from build123d import *

# Parameters (mm, degrees)
F1_DEPTH = 30
F0_R     = 2
F2_DEPTH = 5


with BuildPart() as f1:
    # F0 (on Front) → F1 (new body)
    with BuildSketch(Plane.XZ):
        with BuildLine():
            ThreePointArc((-22.7745900685, 10.3110643104), (0, 25), (22.7745900685, 10.3110643104))
            Line((22.7745900685, 10.3110643104), (28.1723615053, 10.3110643104))
            ThreePointArc((28.1723615053, 10.3110643104), (0, 30), (-28.1723615053, 10.3110643104))
            Line((-28.1723615053, 10.3110643104), (-22.7745900685, 10.3110643104))
        make_face()
        with BuildLine():
            Line((28.1723615053, -10.3110643104), (22.7745900685, -10.3110643104))
            ThreePointArc((22.7745900685, -10.3110643104), (0, -25), (-22.7745900685, -10.3110643104))
            Line((-22.7745900685, -10.3110643104), (-28.1723615053, -10.3110643104))
            ThreePointArc((-28.1723615053, -10.3110643104), (0, -30), (28.1723615053, -10.3110643104))
        make_face()
        with BuildLine():
            ThreePointArc((-22.7745900685, -10.3110643104), (-25, 0), (-22.7745900685, 10.3110643104))
            Line((-22.7745900685, 10.3110643104), (-28.1723615053, 10.3110643104))
            ThreePointArc((-28.1723615053, 10.3110643104), (-30, 0), (-28.1723615053, -10.3110643104))
            Line((-28.1723615053, -10.3110643104), (-22.7745900685, -10.3110643104))
        make_face()
        with BuildLine():
            ThreePointArc((22.7745900685, 10.3110643104), (24.4373152342, 5.2742415705), (25, 0))
            ThreePointArc((25, 0), (24.4373152342, -5.2742415705), (22.7745900685, -10.3110643104))
            Line((22.7745900685, -10.3110643104), (28.1723615053, -10.3110643104))
            ThreePointArc((28.1723615053, -10.3110643104), (29.5395569124, -5.2358931826), (30, 0))
            ThreePointArc((30, 0), (29.5395569124, 5.2358931826), (28.1723615053, 10.3110643104))
            Line((28.1723615053, 10.3110643104), (22.7745900685, 10.3110643104))
        make_face()
    extrude(amount=F1_DEPTH)

    # F0 (on Front) → F2 (join)
    with BuildSketch(Plane.XZ):
        with BuildLine():
            ThreePointArc((-28.1723615053, -10.3110643104), (-30, 0), (-28.1723615053, 10.3110643104))
            Line((-28.1723615053, 10.3110643104), (-33.4467031677, 10.3110643104))
            ThreePointArc((-33.4467031677, 10.3110643104), (-35, 0), (-33.4467031677, -10.3110643104))
            Line((-33.4467031677, -10.3110643104), (-28.1723615053, -10.3110643104))
        make_face()
        with BuildLine():
            ThreePointArc((-28.1723615053, 10.3110643104), (0, 30), (28.1723615053, 10.3110643104))
            Line((28.1723615053, 10.3110643104), (33.4467031677, 10.3110643104))
            ThreePointArc((33.4467031677, 10.3110643104), (0, 35), (-33.4467031677, 10.3110643104))
            Line((-33.4467031677, 10.3110643104), (-28.1723615053, 10.3110643104))
        make_face()
        with BuildLine():
            Line((33.4467031677, 10.3110643104), (28.1723615053, 10.3110643104))
            ThreePointArc((28.1723615053, 10.3110643104), (29.5395569124, 5.2358931826), (30, 0))
            ThreePointArc((30, 0), (29.5395569124, -5.2358931826), (28.1723615053, -10.3110643104))
            Line((28.1723615053, -10.3110643104), (33.4467031677, -10.3110643104))
            ThreePointArc((33.4467031677, -10.3110643104), (34.60949733, -5.2137025774), (35, 0))
            ThreePointArc((35, 0), (34.60949733, 5.2137025774), (33.4467031677, 10.3110643104))
        make_face()
        with BuildLine():
            Line((33.4467031677, -10.3110643104), (28.1723615053, -10.3110643104))
            ThreePointArc((28.1723615053, -10.3110643104), (0, -30), (-28.1723615053, -10.3110643104))
            Line((-28.1723615053, -10.3110643104), (-33.4467031677, -10.3110643104))
            ThreePointArc((-33.4467031677, -10.3110643104), (0, -35), (33.4467031677, -10.3110643104))
        make_face()
        with BuildLine():
            ThreePointArc((-33.4467031677, -10.3110643104), (-35, 0), (-33.4467031677, 10.3110643104))
            Line((-33.4467031677, 10.3110643104), (-46.3196326792, 10.3110643104))
            ThreePointArc((-46.3196326792, 10.3110643104), (-49.8551665852, 8.8465982163), (-51.3196326792, 5.3110643104))
            Line((-51.3196326792, 5.3110643104), (-51.3196326792, -5.3110643104))
            ThreePointArc((-51.3196326792, -5.3110643104), (-49.8551665852, -8.8465982163), (-46.3196326792, -10.3110643104))
            Line((-46.3196326792, -10.3110643104), (-33.4467031677, -10.3110643104))
        make_face()
        with Locations((-43.3196326792, 0)):
            Circle(F0_R, mode=Mode.SUBTRACT)
        with BuildLine():
            Line((46.3196326792, 10.3110643104), (33.4467031677, 10.3110643104))
            ThreePointArc((33.4467031677, 10.3110643104), (34.60949733, 5.2137025774), (35, 0))
            ThreePointArc((35, 0), (34.60949733, -5.2137025774), (33.4467031677, -10.3110643104))
            Line((33.4467031677, -10.3110643104), (46.3196326792, -10.3110643104))
            ThreePointArc((46.3196326792, -10.3110643104), (49.8551665852, -8.8465982163), (51.3196326792, -5.3110643104))
            Line((51.3196326792, -5.3110643104), (51.3196326792, 5.3110643104))
            ThreePointArc((51.3196326792, 5.3110643104), (49.8551665852, 8.8465982163), (46.3196326792, 10.3110643104))
        make_face()
        with Locations((43.3196326792, 0)):
            Circle(F0_R, mode=Mode.SUBTRACT)
    extrude(amount=F2_DEPTH)


solid = f1.part
Verification items for the finished model (mm, model axes). A direction names the side the tool comes from. Coordinates: 2 decimals unless noted, no trailing zeros. Order: outer loops, then holes, each group sorted by start corner. A loop starts at its lowest first (then second) coordinate and runs counter-clockwise, first axis right, second up.
1. Set-up check for faces 1 (the face through (40, -2, 10.311)), 2 (the face through (-40, -2, -10.311)), 3 (the face through (-15.4, -5, 26.1)), 4 (the face through (-40, -2, 10.311)), 5 (the face through (40, -2, -10.311)): record each of +Z, -Z, +X, -X, +Y, -Y from which the full face is reachable in a straight line by a thin tool's end or side.
Results found:
face 1: +Z, +X, +Y, -Y
face 2: -Z, -X, +Y, -Y
face 3: -Y
face 4: +Z, -X, +Y, -Y
face 5: -Z, +X, +Y, -Y
2. Sectioned sample at A-A, the plane y = -15.25. Record the cut outline in (x, z).
Results found:
outline: circle Ø60 at (0, 0); hole circle Ø50 at (0, 0)
3. Release check for a two-part mould opening along X. For faces 6 (the face through (-45.318, -2.465, 0.088)), 7 (the face through (-0.623, -2.465, -34.994)), 8 (the face through (-23, 0, 11)), 9 (the face through (45.167, -2.465, -0.766)) record: +X half, -X half, draft (parallel to the pull), parting line (faces both ways), or undercut.
Results found:
face 6: undercut
face 7: parting line
face 8: draft
face 9: undercut
4. Go/stop test with flat-tipped pins: pin 1 Ø1.5 at (x, y) = (40, -3.5) entering from -Z; pin 2 Ø3 at (x, z) = (16.5, -16.5) entering from -Y (3 decimals); pin 3 Ø8 at (y, z) = (-21, 22.5) entering from +X; pin 4 Ø12 at (x, y) = (-24.5, -18.5) entering from -Z. Record where each tip stops, or that it passes through.
Results found:
pin 1: stops at z = -10.31
pin 2: passes through
pin 3: stops at x = 23.62
pin 4: stops at z = -23.62
5. Sectioned sample at C-C, the plane y = -3. Record the cut outline in (x, z), and give its area (3 significant figures).
Results found:
outline: (-51.32, -5.31) arc R5 ccw to (-46.32, -10.31) - (-33.45, -10.31) arc R35 ccw to (33.45, -10.31) - (46.32, -10.31) arc R5 ccw to (51.32, -5.31) - (51.32, 5.31) arc R5 ccw to (46.32, 10.31) - (33.45, 10.31) arc R35 ccw to (-33.45, 10.31) - (-46.32, 10.31) arc R5 ccw to (-51.32, 5.31) - close; hole circle Ø4 at (-43.32, 0); hole circle Ø50 at (0, 0); hole circle Ø4 at (43.32, 0)
area: 2,530 mm2
6. Sectioned sample at D-D, the plane z = 21. Record the cut outline in (x, y), and give its area (3 significant figures).
Results found:
outline: (-28, -5) - (-21.42, -5) - (-21.42, -30) - (-13.56, -30) - (-13.56, 0) - (-28, 0) - close; (13.56, -30) - (21.42, -30) - (21.42, -5) - (28, -5) - (28, 0) - (13.56, 0) - close
area: 537 mm2
7. Sectioned sample at B-B, the plane x = -14.5. Record the cut outline in (y, z).
Results found:
outline: (-30, -26.26) - (-5, -26.26) - (-5, -31.86) - (0, -31.86) - (0, -20.37) - (-30, -20.37) - close; (-30, 20.37) - (0, 20.37) - (0, 31.86) - (-5, 31.86) - (-5, 26.26) - (-30, 26.26) - close
8. Scan lines: line 1 (Z direction, x = 0, y = -18); line 2 (X direction, y = -16.5, z = 1); line 3 (Y direction, x = -29, z = 13.5). Record each from-to range of solid material in increasing order.
Results found:
line 1: z = -30 to -25, 25 to 30
line 2: x = -29.98 to -24.98, 24.98 to 29.98
line 3: y = -5 to 0
